Source: CAD feature listing. Evaluate the final solid. Frame: model axes, mm. A direction names the side the tool comes from. Give positions to 0.01 mm unless a question says otherwise; leave off trailing zeros. Loops run counter-clockwise (first coordinate to the right, second up) from the corner with the lowest first, then second, coordinate; pieces in that order, holes last. Notation, with made-up numbers: (-37, -30.5) - (-29, -30.5) arc R21 ccw to (-29, -19.5) - close; hole circle Ø8 at (59, -10). An arc over 180 degrees is marked (long way). Write each question's results on one line, items separated by ' | '. Start each with the question number.
(1) Cut plane A-A on x = 0. Return the cut outline in (y, z).
(2) Contact query for flat-ended pins moving along their axis: pin 1 (12 mm diameter, centred on x = -51, y = -6.5, fed in from +Z); pin 2 (3 mm diameter, centred on x = 57.5, y = -20.5, fed in from +Z); pin 3 (4 mm diameter, centred on x = 30, y = -9, fed in from +Z); pin 4 (3 mm diameter, centred on x = -8.5, z = -31, fed in from -Y). Output: stop coordinate, or through.
(3) Cut plane C-C on z = 0. Return the cut outline in (x, y).
(4) Pull-direction query (X, two-part tool) for faces 3 (the flat face through (-1, 0, 18)), 4 (the cylindrical face through (-4.853, -12.878, 15.025)), 5 (the cylindrical face through (-60.47, -12.522, -46.367)), 6 (the cylindrical face through (-19.07, -12.878, -58.915)); classes: pulls with the +X half, pulls with the -X half, needs draft (parallel to the pull), parting line crosses it, or undercut.
(5) Cut plane B-B on y = -17.25. Return the cut outline in (x, z) (1 decimal).
(6) Reachability of faces 1 (the flat face through (-1, -25.4, 18)), 2 (the cylindrical face through (-60.72, -12.88, -12.57)) from +Z, -Z, +X, -X, +Y, -Y: full face, straight path, thin tool, end or side. Return the list, or none.
(7) Material intervals for line 1 along X through (y, z) = (-23, 17); line 2 along Z through (x, y) = (28.5, -15); line 3 along X through (y, z) = (-9.75, 8), sorted ascending. Write a range as [from, to].
from build123d import *

# Parameters (mm, degrees)
F0_R     = 76.2
F1_DEPTH = 25.4
F3_DEPTH = 25.4


with BuildPart() as f1:
    # F0 (on Front) → F1 (new body)
    with BuildSketch(Plane.XZ):
        Circle(F0_R)
    extrude(amount=F1_DEPTH)

    # F2 (on face) → F3 (cut)
    with BuildSketch(Plane.XZ.offset(25.4)):
        with BuildLine():
            ThreePointArc((16.450121, 34.365732), (-5.247361, 14.883619), (-34.365732, 16.450121))
            Line((-34.365732, 16.450121), (-52.494522, 25.127975))
            ThreePointArc((-52.494522, 25.127975), (-56.583872, 25.258794), (-59.443339, 22.332475))
            ThreePointArc((-59.443339, 22.332475), (-63.133498, 6.812595), (-62.839166, -9.137244))
            ThreePointArc((-62.839166, -9.137244), (-60.6698, -12.606212), (-56.64668, -13.350792))
            Line((-56.64668, -13.350792), (-37.083957, -8.740145))
            ThreePointArc((-37.083957, -8.740145), (-16.812801, -15.096171), (-12.66825, -35.932234))
            Line((-12.66825, -35.932234), (-19.351072, -54.887394))
            ThreePointArc((-19.351072, -54.887394), (-19.04241, -58.967176), (-15.826203, -61.496189))
            ThreePointArc((-15.826203, -61.496189), (21.11375, -59.887057), (50.895007, -37.972993))
            ThreePointArc((50.895007, -37.972993), (51.813965, -33.986089), (49.495687, -30.614816))
            Line((49.495687, -30.614816), (32.402533, -20.042102))
            ThreePointArc((32.402533, -20.042102), (22.56305, -1.213841), (34.365732, 16.450121))
            Line((34.365732, 16.450121), (52.494522, 25.127975))
            ThreePointArc((52.494522, 25.127975), (55.161107, 28.231073), (54.675188, 32.293557))
            ThreePointArc((54.675188, 32.293557), (44.901281, 44.901281), (32.293557, 54.675188))
            ThreePointArc((32.293557, 54.675188), (28.231073, 55.161107), (25.127975, 52.494522))
            Line((25.127975, 52.494522), (16.450121, 34.365732))
        make_face()
    extrude(amount=-F3_DEPTH, mode=Mode.SUBTRACT)


solid = f1.part
Ans:
1) outline: (-25.4, -76.2) - (0, -76.2) - (0, -63.5) - (-25.4, -63.5) - close; (-25.4, 17.19) - (0, 17.19) - (0, 76.2) - (-25.4, 76.2) - close
2) pin 1: z = 61.49 | pin 2: z = 51.68 | pin 3: z = 70.87 | pin 4: through
3) outline: (-76.2, -25.4) - (-63.5, -25.4) - (-63.5, 0) - (-76.2, 0) - close; (22.66, -25.4) - (76.2, -25.4) - (76.2, 0) - (22.66, 0) - close
4) face 3: needs draft | face 4: undercut | face 5: parting line crosses it | face 6: undercut
5) outline: circle Ø152.4 at (0, 0); hole (-62.8, -9.1) arc R5.1 ccw to (-56.6, -13.4) - (-37.1, -8.7) arc R20.8 cw to (-12.7, -35.9) - (-19.4, -54.9) arc R5.1 ccw to (-15.8, -61.5) arc R63.5 ccw to (50.9, -38) arc R5.1 ccw to (49.5, -30.6) - (32.4, -20) arc R20.8 cw to (34.4, 16.5) - (52.5, 25.1) arc R5.1 ccw to (54.7, 32.3) arc R63.5 ccw to (32.3, 54.7) arc R5.1 ccw to (25.1, 52.5) - (16.5, 34.4) arc R38.1 cw to (-34.4, 16.5) - (-52.5, 25.1) arc R5.1 ccw to (-59.4, 22.3) arc R63.5 ccw to start
6) face 1: +Z, -Z, +X, -X, -Y | face 2: +Y, -Y
7) line 1: [-74.28, -61.18], [-35.51, -0.36], [35.51, 74.28] | line 2: [-70.67, -56.75], [-16.92, 12.26], [55.23, 70.67] | line 3: [-75.78, -62.99], [25.28, 75.78]
